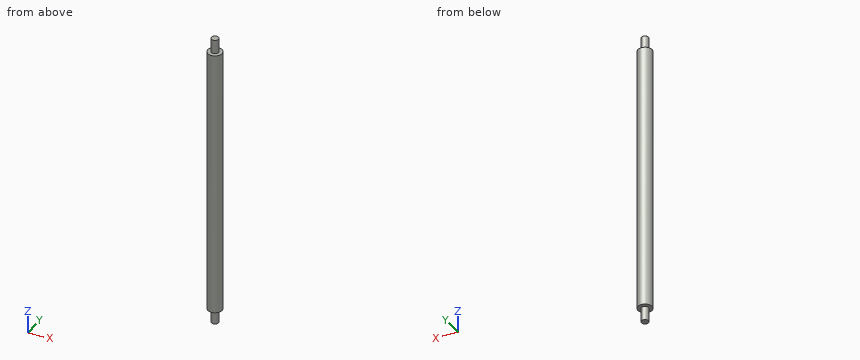
Solid Edge part; units mm, degrees
sketch "Sketch1" plane through (0, 0, 0) normal (0, 0, 1) x (1, 0, 0)
  circle A0 centre (0, 0) radius 1.25
extrude "Protrusion1" add sketch "Sketch1" along normal mid plane 48
sketch "Sketch2" plane through (0, 0, 24) normal (0, 0, 1) x (1, 0, 0)
  circle A0 centre (0, 0) radius 0.625
extrude "Protrusion2" add sketch "Sketch2" along normal up to surface (2.5 mm away)
mirror "Mirror1" about plane through (0, 0, 0) normal (0, 0, 1) of "Protrusion2"
CAD build for the part. Positions are in the model's coordinates, mm. Round coordinates to 2 decimals unless told otherwise and drop trailing zeros. Write each loop counter-clockwise with the first axis right and the second up, starting at its lowest first coordinate (ties: lowest second). Pieces come first, ordered by that corner, then holes. Notation, with made-up numbers: M 17.5,-38.75 L 46.5,-38.75 A13 cw 46.5,-15.75 Z; hole C 13,71.25 d8. An arc over 180 degrees is marked long. Put each result on its own line as item: value. Start each with the question number.
1) Saw through at A-A, the plane x = 0. Write the cut outline in (y, z) (3 decimals), and give its area (3 significant figures).
2) Saw through at C-C, the plane z = -23. Write the cut outline in (x, y), and give its area (3 significant figures).
3) Pin check, flat tip, straight feed: pin 1 Ø1.5 at (y, z) = (-1, 17.5) entering from -X. Stop position of the tip, or through.
4) Drill centre lines: probe 1 along Z at (x, y) = (0.8, 0.5); probe 2 along X at (y, z) = (0.05, -4.5). Where is each one in solid material? Low to high. Write a range as [from, to].
Resolved:
1. outline: M -1.25,-24 L -0.625,-24 L -0.625,-26.5 L 0.625,-26.5 L 0.625,-24 L 1.25,-24 L 1.25,24 L 0.625,24 L 0.625,26.5 L -0.625,26.5 L -0.625,24 L -1.25,24 Z
1. area: 126 mm²
2. outline: C 0,0 d2.5
2. area: 4.91 mm²
3. pin 1: x = -1.22
4. probe 1: [-24, 24]
4. probe 2: [-1.25, 1.25]
